```python
from build123d import *

# Parameters (mm, degrees)
F0_W     = 457.2
F0_H     = 304.8
F1_DEPTH = 9.525
F2_W     = 19.05
F2_H     = 19.05
F3_DEPTH = 19.05
F4_W     = 19.05
F4_H     = 19.05
F5_DEPTH = 19.05


with BuildPart() as f1:
    # F0 (on Front) → F1 (new body, symmetric)
    with BuildSketch(Plane.XZ):
        Rectangle(F0_W, F0_H)
    extrude(amount=F1_DEPTH, both=True)

    # F2 (on face) → F3 (cut)
    with BuildSketch(Plane(origin=(-228.6, 0, 0), x_dir=(0, -1, 0), z_dir=(-1, 0, 0))):
        with Locations((0, 142.875)):
            Rectangle(F2_W, F2_H)
        with Locations((0, 47.625)):
            Rectangle(F2_W, F2_H)
        with Locations((0, -47.625)):
            Rectangle(F2_W, F2_H)
        with Locations((0, -142.875)):
            Rectangle(F2_W, F2_H)
    extrude(amount=-F3_DEPTH, mode=Mode.SUBTRACT)

    # F4 (on face) → F5 (cut)
    with BuildSketch(Plane.YZ.offset(228.6)):
        with Locations((0, 142.875)):
            Rectangle(F4_W, F4_H)
        with Locations((0, 47.625)):
            Rectangle(F4_W, F4_H)
        with Locations((0, -47.625)):
            Rectangle(F4_W, F4_H)
        with Locations((0, -142.875)):
            Rectangle(F4_W, F4_H)
    extrude(amount=-F5_DEPTH, mode=Mode.SUBTRACT)


solid = f1.part
```
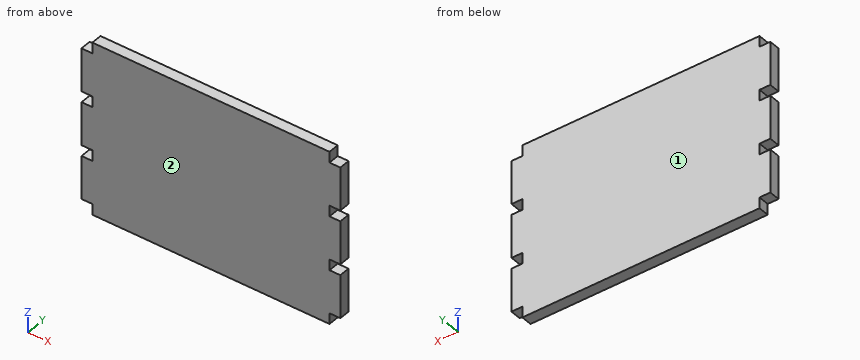
Geometry check sheet. Reference: the model listing, model coordinates, mm. Face numbers are marked on the shaded views. Coordinates: 2 decimals unless noted, no trailing zeros. Write each loop counter-clockwise with the first axis right and the second up, starting at its lowest first coordinate (ties: lowest second). Pieces come first, ordered by that corner, then holes. Notation, with made-up numbers: M 88,17 L 143,17 A14 ccw 143,43 Z; hole C 73.25,-33.5 d1. An arc over 180 degrees is marked long. Answer as a JSON object with one key per item and string values.
1. Section check A-A, the plane y = -2.75. Enter the section's corners in (x, z), plus the area to 3 significant figures.
Answers below:
{"outline": "M -228.6,-133.35 L -209.55,-133.35 L -209.55,-152.4 L 209.55,-152.4 L 209.55,-133.35 L 228.6,-133.35 L 228.6,-57.15 L 209.55,-57.15 L 209.55,-38.1 L 228.6,-38.1 L 228.6,38.1 L 209.55,38.1 L 209.55,57.15 L 228.6,57.15 L 228.6,133.35 L 209.55,133.35 L 209.55,152.4 L -209.55,152.4 L -209.55,133.35 L -228.6,133.35 L -228.6,57.15 L -209.55,57.15 L -209.55,38.1 L -228.6,38.1 L -228.6,-38.1 L -209.55,-38.1 L -209.55,-57.15 L -228.6,-57.15 Z", "area": "136,000 mm²"}
2. Go/stop test with flat-tipped pins: pin 1 Ø9.5 at (x, y) = (-220.5, -2) entering from -Z; pin 2 Ø9.5 at (y, z) = (-3.5, -45) entering from +X; pin 3 Ø1.5 at (y, z) = (-2.5, -55.5) entering from -X. Record where each tip stops, or that it passes through.
Answers below:
{"pin 1": "stops at z = -133.35", "pin 2": "stops at x = 209.55", "pin 3": "stops at x = -209.55"}
3. Draft check along Y on the marked faces 1 and 2. Enter one of: released by +Y, released by -Y, zero draft, split by the parting line, or undercut.
Answers below:
{"face 1": "released by +Y", "face 2": "released by -Y"}
4. Scan line: L1, parallel to X at y = -7.25, z = 140.5. Record every from-to range of solid material in increasing order.
Answers below:
{"L1": "x = -209.55 to 209.55"}
